```python
from build123d import *

# Parameters (mm, degrees)
SKETCH1_W               = 76.19999999999999
SKETCH1_H               = 76.2
BOSS_EXTRUDE1_DEPTH     = 12.7
CUT_EXTRUDE1_DEPTH      = 6.35
SKETCH4_W               = 20.320000000000007
SKETCH4_H               = 20.32
SKETCH4_R               = 5.041900000000002
BOSS_EXTRUDE2_DEPTH     = 12.7
CUT_EXTRUDE2_DEPTH      = 120.21776209944557
CUT_EXTRUDE2_DEPTH_BACK = 120.21776209944557
SKETCH4_3_R             = 5.041900000000002
FILLET2_R               = 9.525
FILLET3_R               = 3.175
CUT_EXTRUDE3_REACH      = 123.23
SKETCH5_R               = 3.174999999999997
SKETCH5_R_2             = 3.174999999999998
SKETCH6_R               = 5.041900000000002
BOSS_EXTRUDE3_DEPTH     = 63.5
CUT_EXTRUDE4_DEPTH      = 9.525
FILLET4_R               = 3.175
FILLET5_R               = 6.35
FILLET6_R               = 2.54
FILLET7_R               = 1.9049999999999998


with BuildPart() as part:
    # Sketch1 → Boss-Extrude1 (new, symmetric)
    with BuildSketch(Plane(origin=(0, 0, 0), x_dir=(1, 0, 0), z_dir=(0, 1, 0))):
        with Locations((38.099999999999994, 38.1)):
            Rectangle(SKETCH1_W, SKETCH1_H)
    extrude(amount=BOSS_EXTRUDE1_DEPTH, both=True)

    # Sketch3 → Cut-Extrude1 (cut, symmetric)
    with BuildSketch(Plane(origin=(0, 0, 0), x_dir=(1, 0, 0), z_dir=(0, 1, 0))):
        Polygon((63.499999999999986, 63.5), (-2.082e-14, 63.5), (0, 0), (63.5, 1.7e-16), align=None)
    extrude(amount=CUT_EXTRUDE1_DEPTH, both=True, mode=Mode.SUBTRACT)

    # Sketch4 → Boss-Extrude2 (add, symmetric)
    with BuildSketch(Plane(origin=(0, 0, 0), x_dir=(1, 0, 0), z_dir=(0, 1, 0))):
        with Locations((73.66, 73.66000000000001)):
            Rectangle(SKETCH4_W, SKETCH4_H)
        with Locations((71.15809999999999, 71.1581)):
            Circle(SKETCH4_R, mode=Mode.SUBTRACT)
    extrude(amount=BOSS_EXTRUDE2_DEPTH, both=True)

    # Sketch4<3> → Cut-Extrude2 (cut, two sides: drawn at the far end of the back side and taken through both)
    with BuildSketch(Plane(origin=(0, 0, 0), x_dir=(1, 0, 0), z_dir=(0, 1, 0)).offset(-CUT_EXTRUDE2_DEPTH_BACK)):
        with Locations(Location((71.15809999999999, 71.1581, 0), (0, 0, 270))):
            Circle(SKETCH4_3_R)
    extrude(amount=CUT_EXTRUDE2_DEPTH + CUT_EXTRUDE2_DEPTH_BACK, mode=Mode.SUBTRACT)

    # Fillet2
    # the kernel refuses this fillet: 9.525 mm, written as the material it adds along each edge
    with BuildSketch(Plane(origin=(63.499999999999986, -12.7, -76.2), x_dir=(-1, 0, 0), z_dir=(0, 1, 0))) as fillet2_piece_1:
        with BuildLine():
            CenterArc((9.332555920003912, -9.525000000000006), FILLET2_R, 90, 78.4630409671845)
            Line((0, -7.6200000000000045), (-0.18665111840007853, -7.5819000000000045))
            ThreePointArc((-0.18665111840007853, -7.5819000000000045), (-0.1905000000000001, -3.8100000000000023), (-0.1905000000000001, 0))
            Line((-0.1905000000000001, 0), (0, 0.1905000000000001))
            Line((0, 0.1905000000000001), (9.332555920003912, 0.1905000000000001))
            Line((9.332555920003912, 0.1905000000000001), (9.332555920003912, 0))
        make_face()
    extrude(amount=25.4)
    with BuildSketch(Plane(origin=(76.19999999999999, 12.7, -63.5), x_dir=(0, 0, 1), z_dir=(0, -1, 0))) as fillet2_piece_2:
        with BuildLine():
            CenterArc((9.332555920003905, -9.525000000000006), FILLET2_R, 90, 78.4630409671845)
            Line((0, -7.6200000000000045), (-0.18665111840007853, -7.5819000000000045))
            ThreePointArc((-0.18665111840007853, -7.5819000000000045), (-0.1905000000000001, -3.8100000000000023), (-0.1905000000000001, 0))
            Line((-0.1905000000000001, 0), (0, 0.1905000000000001))
            Line((0, 0.1905000000000001), (9.332555920003905, 0.1905000000000001))
            Line((9.332555920003905, 0.1905000000000001), (9.332555920003905, 0))
        make_face()
    extrude(amount=25.4)

    # Fillet3
    fillet3_edges = [part.edges().sort_by_distance(p)[0] for p in [
        (83.82, 0, -83.82000000000001),
    ]]
    fillet(fillet3_edges, radius=FILLET3_R)

    # Sketch5 → Cut-Extrude3 (cut, up to next)
    with BuildSketch(Plane(origin=(0, 12.7, 0), x_dir=(1, 0, 0), z_dir=(0, 1, 0)), mode=Mode.PRIVATE) as cut_extrude3_sk1:
        with Locations(Location((19.050000000000004, 50.800000000000004, 0), (0, 0, 270))):
            Circle(SKETCH5_R)
    cut_extrude3_tool1 = extrude(cut_extrude3_sk1.sketch, amount=-CUT_EXTRUDE3_REACH, mode=Mode.PRIVATE) & part.part
    # Sketch5 → Cut-Extrude3 (cut, up to next)
    with BuildSketch(Plane(origin=(0, 12.7, 0), x_dir=(1, 0, 0), z_dir=(0, 1, 0)), mode=Mode.PRIVATE) as cut_extrude3_sk2:
        with Locations(Location((50.79999999999999, 19.05, 0), (0, 0, 270))):
            Circle(SKETCH5_R_2)
    cut_extrude3_tool2 = extrude(cut_extrude3_sk2.sketch, amount=-CUT_EXTRUDE3_REACH, mode=Mode.PRIVATE) & part.part
    add(cut_extrude3_tool1.solids().sort_by_distance((19.05, 12.7, -50.8))[0], mode=Mode.SUBTRACT)
    add(cut_extrude3_tool2.solids().sort_by_distance((50.8, 12.7, -19.05))[0], mode=Mode.SUBTRACT)

    # Sketch6 → Boss-Extrude3 (add)
    with BuildSketch(Plane.XZ.offset(12.7)):
        with BuildLine():
            Line((54.16744407999608, -76.2), (54.16744407999608, -54.16744407999608))
            Line((54.16744407999608, -54.16744407999608), (76.19999999999999, -54.16744407999608))
            ThreePointArc((76.19999999999999, -54.16744407999608), (78.34696672547486, -60.191583022616854), (83.82, -63.5))
            Line((83.82, -63.5), (83.82, -80.64500000000001))
            ThreePointArc((83.82, -80.64500000000001), (82.89006403026728, -82.8900640302673), (80.645, -83.82000000000001))
            Line((80.645, -83.82000000000001), (63.499999999999986, -83.82000000000001))
            ThreePointArc((63.499999999999986, -83.82000000000001), (60.19158302261684, -78.34696672547489), (54.16744407999608, -76.2))
        make_face()
        with Locations(Location((71.15809999999999, -71.1581, 0), (0, 0, 90))):
            Circle(SKETCH6_R, mode=Mode.SUBTRACT)
    extrude(amount=BOSS_EXTRUDE3_DEPTH)

    # Sketch7 → Cut-Extrude4 (cut)
    with BuildSketch(Plane.XZ.offset(76.2)):
        Polygon((71.15809999999995, -79.9569181024499), (78.77809999999995, -75.55750905122497), (78.77809999999997, -66.75869094877508), (71.15809999999996, -62.359281897550105), (63.53809999999996, -66.75869094877504), (63.53809999999996, -75.55750905122494), align=None)
    extrude(amount=-CUT_EXTRUDE4_DEPTH, mode=Mode.SUBTRACT)

    # Fillet4
    fillet4_edges = [part.edges().sort_by_distance(p)[0] for p in [
        (54.16744407999608, -44.45, -54.16744407999608),
    ]]
    fillet(fillet4_edges, radius=FILLET4_R)

    # Fillet5
    fillet5_edges = [part.edges().sort_by_distance(p)[0] for p in [
        (66.77122203999804, -12.7, -54.16744407999608),
        (54.16744407999608, -12.7, -66.77122203999804),
        (55.09738004972879, -12.7, -55.09738004972879),
    ]]
    fillet(fillet5_edges, radius=FILLET5_R)

    # Fillet6
    fillet6_edges = [part.edges().sort_by_distance(p)[0] for p in [
        (0, -9.524999999999999, 0),
        (0, 9.524999999999999, 0),
    ]]
    fillet(fillet6_edges, radius=FILLET6_R)

    # Fillet7
    fillet7_edges = [part.edges().sort_by_distance(p)[0] for p in [
        (76.19999999999999, 12.7, -27.083722039998),
        (39.36999999999999, 12.7, 0),
        (0.7439487757861678, 12.7, -0.7439487757861698),
        (83.82, 12.7, -72.0725),
        (72.07249999999999, 12.7, -83.82000000000001),
        (0, 12.7, -39.370000000000005),
        (27.083722039998, 12.7, -76.2),
        (60.191583022616726, 12.7, -78.34696672547484),
        (78.34696672547484, 12.7, -60.191583022616726),
        (82.89006403026728, 12.7, -82.8900640302673),
    ]]
    fillet(fillet7_edges, radius=FILLET7_R)


solid = part.part
```
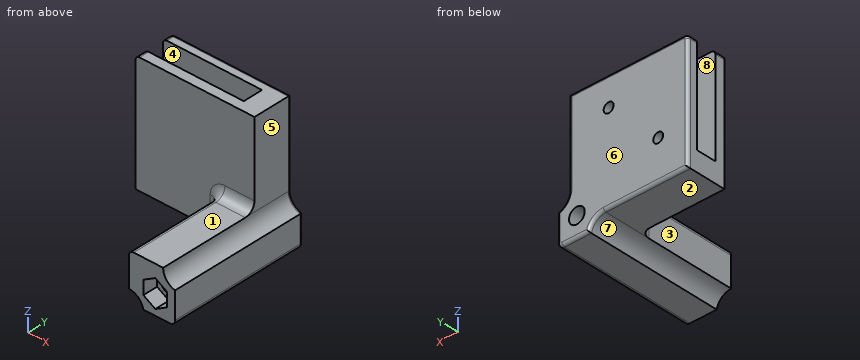
CAD build for the part. Positions are in the model's coordinates, mm. Face numbers are marked on the shaded views. A direction names the side the tool comes from. Give positions to 0.01 mm unless a question says otherwise; leave off trailing zeros. Order: outer loops, then holes, each group sorted by start corner. A loop starts at its lowest first (then second) coordinate and runs counter-clockwise, first axis right, second up. Notation, with made-up numbers: M -10.75,44.25 L 30.25,44.25 A13 cw 30.25,51.25 Z; hole C 57,50 d1. An arc over 180 degrees is marked long. Put each result on its own line as item: value. Start each with the question number.
(1) Saw through at C-C, the plane z = -5. Write the cut outline in (x, y) (3 decimals), then the cut area to 3 significant figures.
(2) Which spindle directions (+Z, -Z, +X, -X, +Y, -Y) get a long thin tool onto all of the face, cutting with end or side? Do the marked faces 1, 2, 3, 4 and 5. Say none if no direction does.
(3) Saw through at B-B, the plane y = -47. Write the cut outline in (x, z) (3 decimals).
(4) Drill centre lines: line 1 along X through (y, z) = (8.5, -19.05) (3 decimals); line 2 along Y through (x, z) = (59, -57); line 3 along Y through (x, z) = (19, -27). Where is each one in solid material? Low to high.
(5) Mould opens along Y. For the marked faces 6, 7 and 8 say: +Y half, -Y half, draft (parallel to the pull), parting line (faces both ways), or undercut.
(6) Saw through at D-D, the plane x = 44. Write the cut outline in (y, z) (3 decimals).
(7) Saw through at A-A, the plane x = 19.05. Write the cut outline in (y, z) (3 decimals).
(8) Flat gauge pins, fed straight in: pin 1 Ø9 at (x, z) = (71.16, -71.16) entering from -Y; pin 2 Ø7.5 at (x, z) = (19.05, -50.8) entering from -Y; pin 3 Ø20.5 at (x, y) = (66, -46.5) entering from +Z; pin 4 Ø15 at (y, z) = (-61, -65.5) entering from -X. Where does each tip first touch, or does it go through?
Check result:
1. outline: M 0,-12.7 L 76.2,-12.7 L 76.2,10.795 A1.905 ccw 74.295,12.7 L 1.905,12.7 A1.905 ccw 0,10.795 L 0,6.35 L 63.5,6.35 L 63.5,-6.35 L 0,-6.35 Z
1. area: 1,130 mm2
2. face 1: +Z, +X, -X, -Y
2. face 2: -Z, -X, +Y, -Y
2. face 3: +Z, -Z, -X, -Y
2. face 4: +Z, -X
2. face 5: +Z, +X, +Y, -Y
3. outline: M 54.167,-76.2 A9.525 cw 63.5,-83.82 L 80.645,-83.82 A3.175 ccw 83.82,-80.645 L 83.82,-63.5 A9.525 cw 76.2,-54.167 L 57.342,-54.167 A3.175 ccw 54.167,-57.342 Z; hole C 71.158,-71.158 d10.084
4. line 1: x = 0 to 47.625, 53.975 to 76.2
4. line 2: y = -76.2 to -6.35, 6.35 to 12.7
4. line 3: y = -12.7 to -6.35, 6.35 to 12.7
5. face 6: +Y half
5. face 7: draft
5. face 8: undercut
6. outline: M -12.7,-76.2 L 10.795,-76.2 A1.905 ccw 12.7,-74.295 L 12.7,-1.905 A1.905 ccw 10.795,0 L 6.35,0 L 6.35,-63.5 L -6.35,-63.5 L -6.35,0 L -12.7,0 Z
7. outline: M -12.7,-76.2 L 10.795,-76.2 A1.905 ccw 12.7,-74.295 L 12.7,-53.975 L 6.35,-53.975 L 6.35,-63.5 L -6.35,-63.5 L -6.35,0 L -12.7,0 Z; M 6.35,-47.625 L 12.7,-47.625 L 12.7,-1.905 A1.905 ccw 10.795,0 L 6.35,0 Z
8. pin 1: passes through
8. pin 2: stops at y = -12.7
8. pin 3: stops at z = -54.17
8. pin 4: stops at x = 54.17
